Verification items for the finished model (mm, model axes). A direction names the side the tool comes from. Coordinates: 2 decimals unless noted, no trailing zeros. Write each loop counter-clockwise with the first axis right and the second up, starting at its lowest first coordinate (ties: lowest second). Pieces come first, ordered by that corner, then holes. Notation, with made-up numbers: (45, 67.25) -> (76, 67.25) arc R12 cw to (76, 88.25) -> close; hole circle Ø8 at (0, 44.5). An arc over 180 degrees is marked (long way). Write each question's results on one line, items separated by ' | '. Start each with the question number.
from build123d import *

# Parameters (mm, degrees)
SKETCH_1_R      = 11
SKETCH_1_R_2    = 2
EXTRUDE_1_DEPTH = 8


with BuildPart() as part:
    # 草图1 → 凸台-拉伸1 (new body)
    with BuildSketch(Plane(origin=(0, 0, 0), x_dir=(1, 0, 0), z_dir=(0, 1, 0))):
        Polygon((-130, -30), (-30, -30), (-30, -138), (-20, -138), (-20, -130), (-10, -130), (-10, -138), (0, -138), (0, -130), (10, -130), (10, -138), (20, -138), (20, -130), (30, -130), (30, -30), (138, -30), (138, -20), (130, -20), (130, -10), (138, -10), (138, 0), (130, 0), (130, 10), (138, 10), (138, 20), (130, 20), (130, 30), (30, 30), (30, 138), (20, 138), (20, 130), (10, 130), (10, 138), (0, 138), (0, 130), (-10, 130), (-10, 138), (-20, 138), (-20, 130), (-30, 130), (-30, 30), (-138, 30), (-138, 20), (-130, 20), (-130, 10), (-138, 10), (-138, 0), (-130, 0), (-130, -10), (-138, -10), (-138, -20), (-130, -20), align=None)
        Circle(SKETCH_1_R, mode=Mode.SUBTRACT)
        with Locations((-15.5, 15.5)):
            Circle(SKETCH_1_R_2, mode=Mode.SUBTRACT)
        with Locations((15.5, 15.5)):
            Circle(SKETCH_1_R_2, mode=Mode.SUBTRACT)
        with Locations((-15.5, -15.5)):
            Circle(SKETCH_1_R_2, mode=Mode.SUBTRACT)
        with Locations((15.5, -15.5)):
            Circle(SKETCH_1_R_2, mode=Mode.SUBTRACT)
    extrude(amount=EXTRUDE_1_DEPTH)


solid = part.part
1. Depth check by flat-ended pin: pin 1 Ø2.5 at (y, z) = (5, -24.5) entering from +X; pin 2 Ø2.5 at (y, z) = (3, -133.5) entering from -X; pin 3 Ø2.5 at (x, y) = (-99, 5.5) entering from +Z. Enter the tip coordinate at first touch or a pass-through.
2. Material ranges on probe 1 along X at (y, z) = (5.25, -15.5); probe 2 along X at (y, z) = (3.5, 15.5), recorded low to high. Write a range as from..to.
3. Sectioned sample at C-C on z = 88.5. Record the cut outline in (x, y), plus the area to 3 significant figures.
4. Sectioned sample at B-B on x = 63. Record the cut outline in (y, z).
5. Mould release check, pull along X, two halves, no side actions. Record for faces 1 (the flat face through (10, 4, 134)), 2 (the flat face through (10, 4, -134)), 3 (the flat face through (134, 4, -20)), 4 (the flat face through (130, 4, -5)): +X half, -X half, draft (parallel to the pull), parting line (faces both ways), or undercut.
6. Tool access check on faces 5 (the flat face through (0, 4, 134)), 6 (the flat face through (134, 4, 10)), 7 (the flat face through (81, 4, -30)). Record the directions out of +Z, -Z, +X, -X, +Y, -Y that give a thin tool (end or side, any length) a straight path to the whole face; none if there is none.
7. Sectioned sample at A-A on y = 2. State how many separate pieces and enclosed holes the cut face has, plus the area to 3 significant figures.
Computed values:
1) pin 1: stops at x = 130 | pin 2: stops at x = -20 | pin 3: stops at z = 30
2) probe 1: x = -130..-17.5, -13.5..13.5, 17.5..138 | probe 2: x = -138..-17.5, -13.5..13.5, 17.5..130
3) outline: (-30, 0) -> (30, 0) -> (30, 8) -> (-30, 8) -> close | area: 480 mm^2
4) outline: (0, -30) -> (8, -30) -> (8, 30) -> (0, 30) -> close
5) face 1: undercut | face 2: undercut | face 3: draft | face 4: +X half
6) face 5: +Z, +Y, -Y | face 6: +X, +Y, -Y | face 7: -Z, +X, +Y, -Y
7) separate pieces: 1 | enclosed holes: 5 | area: 28,100 mm^2
